Here's how the part is built. I have some questions about the finished solid (model axes, mm). A direction names the side the tool comes from. Round coordinates to 2 decimals unless told otherwise and drop trailing zeros. Order: outer loops, then holes, each group sorted by start corner. A loop starts at its lowest first (then second) coordinate and runs counter-clockwise, first axis right, second up.
```python
from build123d import *

# Parameters (mm, degrees)
PAD_DEPTH       = 9.525
SKETCH001_W     = 50.8
SKETCH001_H     = 50.8
POCKET_DEPTH    = 3.175
SKETCH002_W     = 50.8
SKETCH002_H     = 50.8
POCKET001_DEPTH = 3.175
POCKET002_DEPTH = 3.175
SKETCH004_W     = 0.79375
SKETCH004_H     = 0.5
SKETCH004_W_2   = 1.5875
SKETCH004_W_3   = 2.38125
SKETCH004_W_4   = 4.7625
POCKET003_DEPTH = 3.175
POCKET004_DEPTH = 0.5
POCKET005_DEPTH = 0.5


with BuildPart() as part:
    # Sketch → Pad (new body)
    with BuildSketch(Plane.XZ):
        Polygon((0, 0), (50.8, 0), (0, 50.8), align=None)
    extrude(amount=PAD_DEPTH)

    # Sketch001 (on Face5 of Pad) → Pocket (cut)
    with BuildSketch(Plane.XZ.offset(9.525)):
        with Locations((25.4, 28.575)):
            Rectangle(SKETCH001_W, SKETCH001_H)
    extrude(amount=-POCKET_DEPTH, mode=Mode.SUBTRACT)

    # Sketch002 (on Face4 of Pocket) → Pocket001 (cut)
    with BuildSketch(Plane(origin=(0, 0, 0), x_dir=(1, 0, 0), z_dir=(0, 1, 0))):
        with Locations((25.4, -28.575)):
            Rectangle(SKETCH002_W, SKETCH002_H)
    extrude(amount=-POCKET001_DEPTH, mode=Mode.SUBTRACT)

    # Sketch003 (on Face7 of Pocket001) → Pocket002 (cut)
    with BuildSketch(Plane.XZ.offset(6.35)):
        Polygon((6.35, 6.35), (26.67, 6.35), (6.35, 26.67), align=None)
        Polygon((6.35, 31.4325), (6.35, 36.195), (36.195, 6.35), (31.4325, 6.35), align=None)
    extrude(amount=-POCKET002_DEPTH, mode=Mode.SUBTRACT)

    # Sketch004 (on Face7 of Pocket002) → Pocket003 (cut)
    with BuildSketch(Plane.XZ.offset(6.35)):
        with Locations((0.896875, 3.175)):
            Rectangle(SKETCH004_W, SKETCH004_H)
        with Locations((1.293865, 6.346028)):
            Rectangle(SKETCH004_W_2, SKETCH004_H)
        with Locations((0.897105, 9.517056)):
            Rectangle(SKETCH004_W, SKETCH004_H)
        with Locations((1.69097, 12.688084)):
            Rectangle(SKETCH004_W_3, SKETCH004_H)
        with Locations((0.897335, 15.859112)):
            Rectangle(SKETCH004_W, SKETCH004_H)
        with Locations((1.294325, 19.03014)):
            Rectangle(SKETCH004_W_2, SKETCH004_H)
        with Locations((0.897565, 22.201168)):
            Rectangle(SKETCH004_W, SKETCH004_H)
        with Locations((2.882055, 25.372196)):
            Rectangle(SKETCH004_W_4, SKETCH004_H)
        with Locations((0.897795, 28.543224)):
            Rectangle(SKETCH004_W, SKETCH004_H)
        with Locations((1.294785, 31.714252)):
            Rectangle(SKETCH004_W_2, SKETCH004_H)
        with Locations((0.898025, 34.88528)):
            Rectangle(SKETCH004_W, SKETCH004_H)
        with Locations((1.69189, 38.056308)):
            Rectangle(SKETCH004_W_3, SKETCH004_H)
        with Locations((0.898255, 41.227336)):
            Rectangle(SKETCH004_W, SKETCH004_H)
        with Locations((1.295245, 44.398364)):
            Rectangle(SKETCH004_W_2, SKETCH004_H)
        with Locations((0.898485, 47.569392)):
            Rectangle(SKETCH004_W, SKETCH004_H)
    extrude(amount=-POCKET003_DEPTH, mode=Mode.SUBTRACT)

    # Sketch005 (on Face7 of Pocket003) → Pocket004 (cut)
    with BuildSketch(Plane.XZ.offset(6.35)):
        Polygon((43.954481, 3.845519), (46.713131, 4.086869), (47.625, 3.175), (44.625, 3.175), align=None)
        Polygon((40.63496, 7.16504), (43.185271, 7.614729), (40.064697, 10.735303), (37.698671, 10.101329), align=None)
        Polygon((28.114215, 19.685785), (29.878705, 20.921295), (32.205909, 18.594091), (30.303986, 17.496014), align=None)
        Polygon((25.4, 25.4), (27.622212, 23.177788), (25.990979, 21.809021), (23.9, 23.9), align=None)
        Polygon((23.177788, 27.622212), (21.809021, 25.990979), (19.685785, 28.114215), (20.921295, 29.878705), align=None)
        Polygon((15.201111, 32.598889), (17.496014, 30.303986), (18.594091, 32.205909), (16.155156, 34.644844), align=None)
        Polygon((13.555785, 37.244215), (10.735303, 40.064697), (10.101329, 37.698671), (12.755247, 35.044753), align=None)
        Polygon((7.614729, 43.185271), (4.086869, 46.713131), (3.845519, 43.954481), (7.16504, 40.63496), align=None)
        Polygon((32.598889, 15.201111), (34.644844, 16.155156), (37.244215, 13.555785), (35.044753, 12.755247), align=None)
    extrude(amount=-POCKET004_DEPTH, mode=Mode.SUBTRACT)

    # Sketch006 → Pocket005 (cut)
    with BuildSketch(Plane(origin=(0, -3.175, 0), x_dir=(1, 0, 0), z_dir=(0, 1, 0))):
        Polygon((43.185271, -7.614729), (40.064697, -10.735303), (37.698671, -10.101329), (40.63496, -7.16504), align=None)
        Polygon((37.244215, -13.555785), (34.644844, -16.155156), (32.598889, -15.201111), (35.044753, -12.755247), align=None)
        Polygon((32.205909, -18.594091), (29.878705, -20.921295), (28.114215, -19.685785), (30.303986, -17.496014), align=None)
        Polygon((27.622212, -23.177788), (25.4, -25.4), (23.9, -23.9), (25.990979, -21.809021), align=None)
        Polygon((23.177788, -27.622212), (20.921295, -29.878705), (19.685785, -28.114215), (21.809021, -25.990979), align=None)
        Polygon((17.496014, -30.303986), (18.594091, -32.205909), (16.155156, -34.644844), (15.201111, -32.598889), align=None)
        Polygon((13.555785, -37.244215), (10.735303, -40.064697), (10.101329, -37.698671), (12.755247, -35.044753), align=None)
        Polygon((7.614729, -43.185271), (4.086869, -46.713131), (3.845519, -43.954481), (7.16504, -40.63496), align=None)
        Polygon((46.713131, -4.086869), (43.954481, -3.845519), (44.625, -3.175), (47.625, -3.175), align=None)
    extrude(amount=-POCKET005_DEPTH, mode=Mode.SUBTRACT)


solid = part.part
```
1. If we mould it in two halves opening along X, with no side actions, what happens to faces 5 (the flat face through (29.2, -6.1, 18.6)), 6 (the flat face through (29.3, -5.1, 21.5)), 7 (the flat face through (18, -3.175, 16))? For each: released by +X, released by -X, zero draft, split by the parting line, or undercut.
Evaluation:
face 5: undercut
face 6: released by +X
face 7: zero draft
2. If we section it at A-A, the plane x = 12: State how many separate pieces and enclosed holes the cut face has, and give its area (3 significant figures).
Evaluation:
separate pieces: 3
enclosed holes: 0
area: 78.7 mm2
3. On a 3-axis mill with a long thin cutter (end or side, diameter ignored), from which of +Z, -Z, +X, -X, +Y, -Y can I reach the whole of each face in a straight line? I mean faces 1 (the flat face through (20.7, -3.4, 27.1)), 2 (the flat face through (3, -5, 25.622)), 3 (the flat face through (33.8, -6.1, 14)), 4 (the flat face through (18.037, -3.422, 31.242)). Say none if no direction works.
Evaluation:
face 1: +Y
face 2: +Y, -Y
face 3: -Y
face 4: +Z, +Y
4. If we section it at D-D, the plane x = 39: Write out the boundary of the cut face in (y, z) (3 decimals), and give its area (3 significant figures).
Evaluation:
outline: (-9.525, 0) - (0, 0) - (0, 3.175) - (-3.175, 3.175) - (-3.175, 8.8) - (-3.675, 8.8) - (-3.675, 10.45) - (-3.175, 10.45) - (-3.175, 11.8) - (-6.35, 11.8) - (-6.35, 10.45) - (-5.85, 10.45) - (-5.85, 8.8) - (-6.35, 8.8) - (-6.35, 3.175) - (-9.525, 3.175) - close
area: 56.0 mm2
5. If we section it at C-C, the plane y = -2.5: Write out the boundary of the cut face in (x, z) (3 decimals).
Evaluation:
outline: (0, 0) - (50.8, 0) - (47.625, 3.175) - (0, 3.175) - close
6. If we section it at B-B, the plane z = 45.5: Write out the boundary of the cut face in (x, y) (3 decimals).
Evaluation:
outline: (0, -6.35) - (3.981, -6.35) - (3.981, -5.85) - (5.3, -5.85) - (5.3, -3.675) - (3.981, -3.675) - (3.981, -3.175) - (0, -3.175) - close
7. I'm going to push flat-ended pins straight in: P1, Ø5, axis at y = -7, z = 26, coming from the +X side; P2, Ø3.5, axis at y = -5.5, z = 20, coming from the +X side; P3, Ø5, axis at x = 9, z = 36.5, coming from the -Y side. Where does each tip first touch, or does it pass through?
Evaluation:
P1: stops at x = 27.02
P2: stops at x = 32.55
P3: stops at y = -6.35
8. I need wall thicknesses on probe 1 along Z at (x, y) = (25.5, -0.5) (3 decimals); probe 2 along Y at (x, z) = (2.5, 23) (3 decimals); probe 3 along X at (y, z) = (-4.25, 30.5) (1 decimal). Which ranges of each line are inside material? Lowest first, please.
Evaluation:
probe 1: z = 0 to 3.175
probe 2: y = -6.35 to -3.175
probe 3: x = 0 to 7.3, 12 to 20.3
